Check sheet for the modelled part. Datum: model origin and axes. Units: mm. A direction names the side the tool comes from. Give positions to 0.01 mm unless a question says otherwise; leave off trailing zeros. Write each loop counter-clockwise with the first axis right and the second up, starting at its lowest first coordinate (ties: lowest second). Pieces come first, ordered by that corner, then holes. Notation, with made-up numbers: (4.25, -12) - (44.25, -12) arc R35 ccw to (44.25, 23) - close; hole circle Ø5 at (57.25, 40.25). An arc over 180 degrees is marked (long way). Return JSON: item names as keys, results as strings. Group by question number.
Solid Edge part; units mm, degrees
sketch "Sketch1" plane through (0, 0, 0) normal (0, -1, 0) x (1, 0, 0)
  circle A0 centre (0, 0) radius 18.5
extrude "Protrusion1" add sketch "Sketch1" against normal blind 47
sketch "Sketch2" plane through (0, 47, 0) normal (0, 1, 0) x (1, 0, 0)
  circle A0 centre (0, 6.999) radius 6
extrude "ExtrudedProtrusion_2" add sketch "Sketch2" along normal blind 6
sketch "Sketch3" plane through (0, 47, 0) normal (0, 1, 0) x (1, 0, 0)
  circle A0 centre (0, 6.999) radius 3
extrude "ExtrudedProtrusion_3" add sketch "Sketch3" along normal blind 21
chamfer "Chamfer_1" distance 0.5 angle 45 1 edges at (-3, 68, -6.999)
sketch "Sketch4" plane through (0, 0, 0) normal (-1, 0, 0) x (0, -1, 0)
  line L0 (0, 16.3) -> (-23, 16.3)
  line L1 (-23, 16.3) -> (-23, 18.5)
  line L2 (-23, 18.5) -> (0, 18.5)
  line L3 (0, 18.5) -> (0, 16.3)
  dimension "D1" = 23
revolve "RevolvedCutout1" cut sketch "Sketch4" angle 360 about axis through (0, 0, 0) along (0, 1, 0)
Item 1: Section check B-B on z = 0. Record the cut outline in (x, y), plus the area to 3 significant figures.
Item 2: Section check A-A on x = 0. Record the cut outline in (y, z), plus the area to 3 significant figures.
Item 3: Material ranges on line 1 along Y through (x, z) = (4.5, -15.5); line 2 along Y through (x, z) = (15, 6.5); line 3 along X through (y, z) = (17, -8), recorded low to high. Write a range as from..to.
Item 4: Depth check by flat-ended pin: pin 1 (2 mm diameter, centred on y = 37, z = -13, fed in from +X); pin 2 (5 mm diameter, centred on y = 17, z = -4.5, fed in from -X); pin 3 (1.5 mm diameter, centred on x = 7.5, y = 33, fed in from -Z). Enter the tip coordinate at first touch or a pass-through.
Item 5: Section check C-C on y = 19. Record the cut outline in (x, z).
Item 6: Section check D-D on x = -9. Record the cut outline in (y, z), plus the area to 3 significant figures.
Item 7: Access from +Z, -Z, +X, -X, +Y, -Y to the whole of each face (thin tool, end or side, straight path). Record for faces 1 (the face through (-16.4, 23, 1.3)), 2 (the face through (-3, 60, -7)), 3 (the face through (0, 0, 0)).
Reply:
{
 "1": {"outline": "(-18.5, 23) - (-16.3, 23) - (-16.3, 0) - (16.3, 0) - (16.3, 23) - (18.5, 23) - (18.5, 47) - (-18.5, 47) - close", "area": "1,640 mm²"},
 "2": {"outline": "(0, -16.3) - (23, -16.3) - (23, -18.5) - (47, -18.5) - (47, -13) - (53, -13) - (53, -10) - (67.5, -10) - (68, -9.5) - (68, -4.5) - (67.5, -4) - (53, -4) - (53, -1) - (47, -1) - (47, 18.5) - (23, 18.5) - (23, 16.3) - (0, 16.3) - close", "area": "1,800 mm²"},
 "3": {"line 1": "0..47", "line 2": "23..47", "line 3": "-14.2..14.2"},
 "4": {"pin 1": "x = 14.08", "pin 2": "x = -16.18", "pin 3": "z = -17.22"},
 "5": {"outline": "circle Ø32.6 at (0, 0)"},
 "6": {"outline": "(0, -13.59) - (23, -13.59) - (23, -16.16) - (47, -16.16) - (47, 16.16) - (23, 16.16) - (23, 13.59) - (0, 13.59) - close", "area": "1,400 mm²"},
 "7": {"face 1": "-Y", "face 2": "+Y", "face 3": "+Z, -Z, +X, -X, -Y"}
}
